The figure shows three views and two pictorial views of one solid part (mm, origin at its lowest corner). Answer the questions. A direction names the side the tool comes from. Coordinates: 2 decimals unless noted, no trailing zeros. Write each loop counter-clockwise with the first axis right and the second up, starting at its lowest first coordinate (ties: lowest second). Pieces come first, ordered by that corner, then holes.
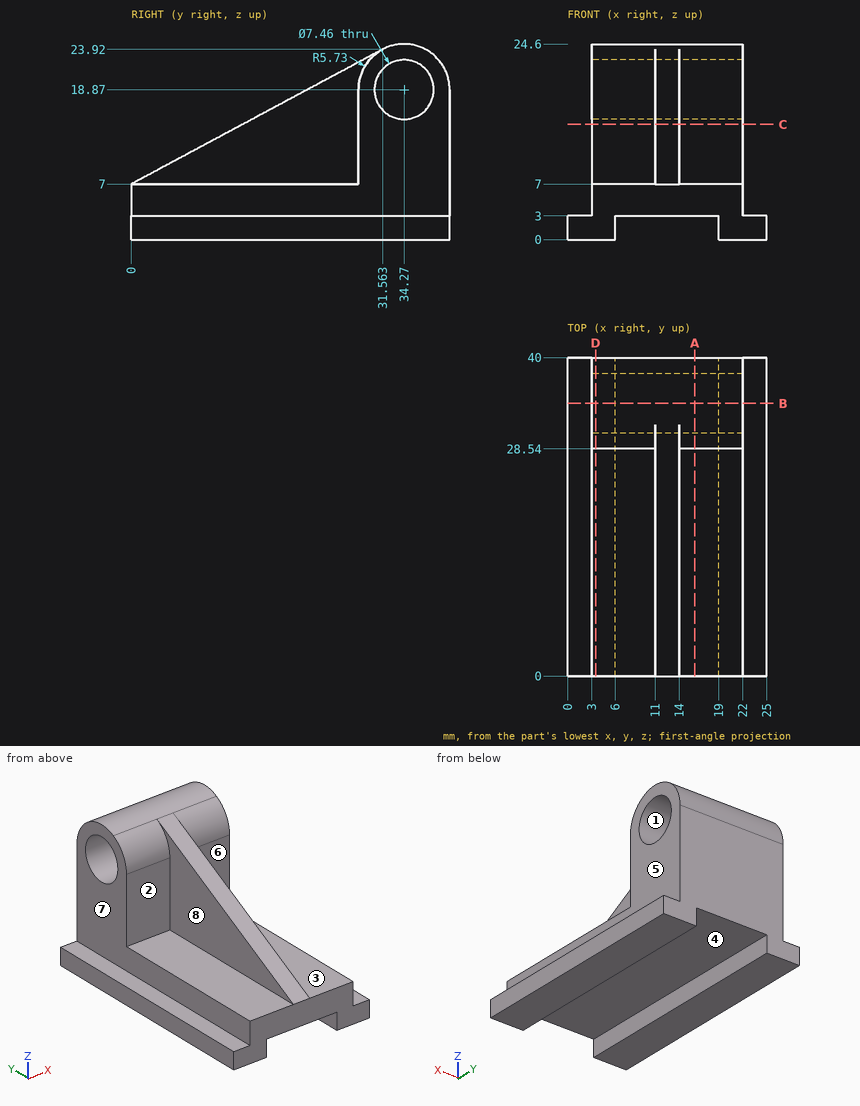
Item 1: The part is cut by section B-B (y = 34.27). Give the vertices of the cut face in (x, z), and give its area (3 significant figures).
Item 2: The part is cut by section A-A (x = 16). Give the vertices of the cut face in (y, z), and give its area (3 significant figures).
Item 3: The part is cut by section D-D (x = 3.5). Give the vertices of the cut face in (y, z).
Item 4: The part is cut by section C-C (z = 14.5). Give the vertices of the cut face in (x, y).
Item 5: For the marked faces 4, 5, 6, 7 and 8, determine the directions among +Z, -Z, +X, -X, +Y, -Y from which every point of the face is accessible in a straight line to the end or side of a thin tool.
Item 6: Determine the mould class of the marked faces 1, 2 and 3 for opening direction Z: +Z half, -Z half, draft (parallel to the pull), parting line (faces both ways), or undercut.
Item 7: Given pin 1 (2 mm diameter, centred on x = 12.5, y = 21, fed in from +Z); pin 2 (6.5 mm diameter, centred on x = 18, z = 15.5, fed in from -Y); pin 3 (6.5 mm diameter, centred on x = 19.5, y = 15.5, fed in from +Z), each flat-ended and moving along its own axis, determine where each tip first touches the part or whether it passes through.
Item 8: Find the intervals of material crossed by probe 1 along X at (y, z) = (6, 2); probe 2 along Z at (x, y) = (9.25, 34.27); probe 3 along X at (y, z) = (29.5, 5), in increasing order.
Answer:
1. outline: (0, 0) - (6, 0) - (6, 3) - (19, 3) - (19, 0) - (25, 0) - (25, 3) - (22, 3) - (22, 15.14) - (3, 15.14) - (3, 3) - (0, 3) - close; (3, 22.6) - (22, 22.6) - (22, 24.6) - (3, 24.6) - close
1. area: 305 mm2
2. outline: (0, 3) - (40, 3) - (40, 18.87) arc R5.73 ccw to (28.54, 18.87) - (28.54, 7) - (0, 7) - close; hole circle Ø7.46 at (34.27, 18.87)
2. area: 304 mm2
3. outline: (0, 0) - (40, 0) - (40, 18.87) arc R5.73 ccw to (28.54, 18.87) - (28.54, 7) - (0, 7) - close; hole circle Ø7.46 at (34.27, 18.87)
4. outline: (3, 28.54) - (11, 28.54) - (11, 13.99) - (14, 13.99) - (14, 28.54) - (22, 28.54) - (22, 40) - (3, 40) - close
5. face 4: -Z, +Y, -Y
5. face 5: +Z, +X, +Y, -Y
5. face 6: +Z, +X, -Y
5. face 7: +Z, -X, +Y, -Y
5. face 8: +Z, -X, -Y
6. face 1: undercut
6. face 2: draft
6. face 3: +Z half
7. pin 1: stops at z = 18.79
7. pin 2: stops at y = 28.54
7. pin 3: stops at z = 7
8. probe 1: x = 0 to 6, 19 to 25
8. probe 2: z = 3 to 15.14, 22.6 to 24.6
8. probe 3: x = 3 to 22
